For this review, take the finished solid that the model builds, in its own axes (mm). A direction names the side the tool comes from. Coordinates: 2 decimals unless noted, no trailing zeros. Write each loop counter-clockwise with the first axis right and the second up, starting at its lowest first coordinate (ties: lowest second). Pieces come first, ordered by that corner, then holes.
```python
from build123d import *

# Parameters (mm, degrees)
SKETCH1_W                      = 54
SKETCH1_H                      = 60
BOSS_EXTRUDE1_DEPTH            = 6
CBORE_FOR_M4_SHCS1_D           = 4.5
CBORE_FOR_M4_SHCS1_DEPTH       = 12.4
CBORE_FOR_M4_SHCS1_CBORE_D     = 8
CBORE_FOR_M4_SHCS1_CBORE_DEPTH = 4
CBORE_FOR_M4_SHCS1_TIP         = 1.351936393
CUT_EXTRUDE1_DEPTH             = 4
FILLET1_SIZE                   = 5
CUT_EXTRUDE2_DEPTH             = 41.804411681
BOSS_EXTRUDE2_START            = -5
SKETCH6_W                      = 14.857864376
SKETCH6_H                      = 14
SKETCH6_R                      = 3
BOSS_EXTRUDE2_DEPTH            = 36
FILLET3_SIZE                   = 5


with BuildPart() as part:
    # Sketch1 → Boss-Extrude1 (new body)
    with BuildSketch(Plane(origin=(0, 0, 0), x_dir=(1, 0, 0), z_dir=(0, 1, 0))):
        Rectangle(SKETCH1_W, SKETCH1_H)
    extrude(amount=BOSS_EXTRUDE1_DEPTH)

    # CBORE for M4 SHCS1
    with Locations(Plane(origin=(0, 6, 0), x_dir=(1, 0, 0), z_dir=(0, 1, 0))):
        with Locations((-22.5, 25.5), (-22.5, -25.5), (22.5, -25.5), (22.5, 25.5)):
            CounterBoreHole(CBORE_FOR_M4_SHCS1_D / 2, CBORE_FOR_M4_SHCS1_CBORE_D / 2, CBORE_FOR_M4_SHCS1_CBORE_DEPTH, depth=CBORE_FOR_M4_SHCS1_DEPTH)
            with Locations((0, 0, -(CBORE_FOR_M4_SHCS1_DEPTH + CBORE_FOR_M4_SHCS1_TIP / 2))):  # 118° drill point
                Cone(0, CBORE_FOR_M4_SHCS1_D / 2, CBORE_FOR_M4_SHCS1_TIP, mode=Mode.SUBTRACT)

    # Sketch4 → Cut-Extrude1 (cut)
    with BuildSketch(Plane(origin=(0, 6, 0), x_dir=(1, 0, 0), z_dir=(0, 1, 0))):
        with BuildLine():
            Line((-22.5, 21.5), (-27, 21.5))
            Line((-27, 21.5), (-27, 30))
            Line((-27, 30), (-18.5, 30))
            Line((-18.5, 30), (-18.5, 25.5))
            ThreePointArc((-18.5, 25.5), (-19.671572875, 22.671572875), (-22.5, 21.5))
        make_face()
        with BuildLine():
            Line((22.5, 21.5), (27, 21.5))
            Line((27, 21.5), (27, 30))
            Line((27, 30), (18.5, 30))
            Line((18.5, 30), (18.5, 25.5))
            ThreePointArc((18.5, 25.5), (19.671572875, 22.671572875), (22.5, 21.5))
        make_face()
        with BuildLine():
            Line((18.5, -30), (18.5, -25.5))
            ThreePointArc((18.5, -25.5), (19.671572875, -22.671572875), (22.5, -21.5))
            Line((22.5, -21.5), (27, -21.5))
            Line((27, -21.5), (27, -30))
            Line((27, -30), (18.5, -30))
        make_face()
        with BuildLine():
            Line((-18.5, -30), (-18.5, -25.5))
            ThreePointArc((-18.5, -25.5), (-19.671572875, -22.671572875), (-22.5, -21.5))
            Line((-22.5, -21.5), (-27, -21.5))
            Line((-27, -21.5), (-27, -30))
            Line((-27, -30), (-18.5, -30))
        make_face()
    extrude(amount=-CUT_EXTRUDE1_DEPTH, mode=Mode.SUBTRACT)

    # Fillet1
    # a fillet whose section is not a circle: 5 mm, written as the material it takes off along each edge
    with BuildSketch(Plane(origin=(27, -12.5, -30), x_dir=(0, 0, 1), z_dir=(0, 1, 0)), Plane(origin=(27, -12.5, 30), x_dir=(-1, 0, 0), z_dir=(0, 1, 0))) as fillet1_piece_1:
        with BuildLine():
            add(Edge.make_bspline([(FILLET1_SIZE, 0), (FILLET1_SIZE * 0.831801948466, 0), (FILLET1_SIZE * 0.663603896932, 0), (FILLET1_SIZE * 0.292893218813, -FILLET1_SIZE * 0.0716919198361), (FILLET1_SIZE * 0.0716919198361, -FILLET1_SIZE * 0.292893218813), (0, -FILLET1_SIZE * 0.663603896932), (0, -FILLET1_SIZE * 0.831801948466), (0, -FILLET1_SIZE)], knots=[0, 0, 0, 0, 0, 0, 0.5, 0.5, 1, 1, 1, 1, 1, 1], degree=5))
            Line((0, -FILLET1_SIZE), (0, 0))
            Line((0, 0), (FILLET1_SIZE, 0))
        make_face()
    extrude(amount=27, mode=Mode.SUBTRACT)
    with BuildSketch(Plane(origin=(-27, -12.5, -30), x_dir=(0, 0, 1), z_dir=(0, 1, 0)), Plane(origin=(-27, -12.5, 30), x_dir=(1, 0, 0), z_dir=(0, 1, 0))) as fillet1_piece_2:
        with BuildLine():
            add(Edge.make_bspline([(FILLET1_SIZE, 0), (FILLET1_SIZE * 0.831801948466, 0), (FILLET1_SIZE * 0.663603896932, 0), (FILLET1_SIZE * 0.292893218813, FILLET1_SIZE * 0.0716919198361), (FILLET1_SIZE * 0.0716919198361, FILLET1_SIZE * 0.292893218813), (0, FILLET1_SIZE * 0.663603896932), (0, FILLET1_SIZE * 0.831801948466), (0, FILLET1_SIZE)], knots=[0, 0, 0, 0, 0, 0, 0.5, 0.5, 1, 1, 1, 1, 1, 1], degree=5))
            Line((0, FILLET1_SIZE), (0, 0))
            Line((0, 0), (FILLET1_SIZE, 0))
        make_face()
    extrude(amount=27, mode=Mode.SUBTRACT)

    # Sketch5 → Cut-Extrude2 (cut, through all)
    with BuildSketch(Plane(origin=(0, 6, 0), x_dir=(1, 0, 0), z_dir=(0, 1, 0))):
        Polygon((-27, 13.5), (-23, 9.5), (-23, -9.5), (-27, -13.5), align=None)
        Polygon((27, 13.5), (23, 9.5), (23, -9.5), (27, -13.5), align=None)
    extrude(amount=-CUT_EXTRUDE2_DEPTH, mode=Mode.SUBTRACT)

    # Fillet2
    # a fillet whose section is not a circle: 5 mm, written as the material it adds along each edge
    with BuildSketch(Plane(origin=(-23, 6, 9.5), x_dir=(-0.7071067811865389, 0, 0.7071067811865561), z_dir=(0, -1, 0)), Plane(origin=(23, 6, 9.5), x_dir=(0, 0, -1), z_dir=(0, -1, 0)), Plane(origin=(23, 6, -9.5), x_dir=(0.707106781186557, 0, -0.7071067811865381), z_dir=(0, -1, 0)), Plane(origin=(-23, 6, -9.5), x_dir=(0, 0, 1), z_dir=(0, -1, 0))) as fillet2_piece_1:
        with BuildLine():
            add(Edge.make_bspline([(2.071067812, 0), (1.691961313, 0), (1.312854813, 0), (0.467093497, 0.07115949), (-0.279967621, 0.380602337), (-0.928328541, 0.928328541), (-1.196397318, 1.196397318), (-1.464466094, 1.464466094)], knots=[0, 0, 0, 0, 0, 0, 0.5, 0.5, 1, 1, 1, 1, 1, 1], degree=5))
            Line((-1.464466094, 1.464466094), (0, 0))
            Line((0, 0), (2.071067812, 0))
        make_face()
    extrude(amount=6)
    # a fillet whose section is not a circle: 5 mm, written as the material it takes off along each edge
    with BuildSketch(Plane(origin=(27, 11.17766953, 13.5), x_dir=(-0.7071067811865385, 0, -0.7071067811865565), z_dir=(0, -1, 0)), Plane(origin=(27, 11.17766953, -13.5), x_dir=(0, 0, -1), z_dir=(0, -1, 0)), Plane(origin=(-27, 11.17766953, 13.5), x_dir=(0, 0, 1), z_dir=(0, -1, 0)), Plane(origin=(-27, 11.17766953, -13.5), x_dir=(0.7071067811865569, 0, 0.707106781186538), z_dir=(0, -1, 0))) as fillet2_2_piece_1:
        with BuildLine():
            add(Edge.make_bspline([(2.071067812, 0), (1.691961313, 0), (1.312854813, 0), (0.467093497, -0.07115949), (-0.279967621, -0.380602337), (-0.928328541, -0.928328541), (-1.196397318, -1.196397318), (-1.464466094, -1.464466094)], knots=[0, 0, 0, 0, 0, 0, 0.5, 0.5, 1, 1, 1, 1, 1, 1], degree=5))
            Line((-1.464466094, -1.464466094), (0, 0))
            Line((0, 0), (2.071067812, 0))
        make_face()
    extrude(amount=16.355339059, mode=Mode.SUBTRACT)

    # Sketch6 → Boss-Extrude2 (add)
    with BuildSketch(Plane.ZY.offset(23).offset(BOSS_EXTRUDE2_START)):
        with Locations((0, 13)):
            Rectangle(SKETCH6_W, SKETCH6_H)
        with Locations((0, 14)):
            Circle(SKETCH6_R, mode=Mode.SUBTRACT)
    extrude(amount=-BOSS_EXTRUDE2_DEPTH)

    # Fillet3
    # a fillet whose section is not a circle: 5 mm, written as the material it takes off along each edge
    with BuildSketch(Plane(origin=(-30.5, 20, -7.428932188), x_dir=(0, -1, 0), z_dir=(1, 0, 0))) as fillet3_piece_1:
        with BuildLine():
            add(Edge.make_bspline([(FILLET3_SIZE, 0), (FILLET3_SIZE * 0.831801948466, 0), (FILLET3_SIZE * 0.663603896932, 0), (FILLET3_SIZE * 0.292893218813, -FILLET3_SIZE * 0.0716919198361), (FILLET3_SIZE * 0.0716919198361, -FILLET3_SIZE * 0.292893218813), (0, -FILLET3_SIZE * 0.663603896932), (0, -FILLET3_SIZE * 0.831801948466), (0, -FILLET3_SIZE)], knots=[0, 0, 0, 0, 0, 0, 0.5, 0.5, 1, 1, 1, 1, 1, 1], degree=5))
            Line((0, -FILLET3_SIZE), (0, 0))
            Line((0, 0), (FILLET3_SIZE, 0))
        make_face()
    extrude(amount=61, mode=Mode.SUBTRACT)
    with BuildSketch(Plane(origin=(-30.5, 20, 7.428932188), x_dir=(0, -1, 0), z_dir=(1, 0, 0))) as fillet3_piece_2:
        with BuildLine():
            add(Edge.make_bspline([(FILLET3_SIZE, 0), (FILLET3_SIZE * 0.831801948466, 0), (FILLET3_SIZE * 0.663603896932, 0), (FILLET3_SIZE * 0.292893218813, FILLET3_SIZE * 0.0716919198361), (FILLET3_SIZE * 0.0716919198361, FILLET3_SIZE * 0.292893218813), (0, FILLET3_SIZE * 0.663603896932), (0, FILLET3_SIZE * 0.831801948466), (0, FILLET3_SIZE)], knots=[0, 0, 0, 0, 0, 0, 0.5, 0.5, 1, 1, 1, 1, 1, 1], degree=5))
            Line((0, FILLET3_SIZE), (0, 0))
            Line((0, 0), (FILLET3_SIZE, 0))
        make_face()
    extrude(amount=61, mode=Mode.SUBTRACT)


solid = part.part
```
Q1. Add section B-B (z = 0). State the section outline as (x, y) points, then the cut area to 3 significant figures.
Ans:
outline: (-23, 0) - (23, 0) - (23, 6) - (18, 6) - (18, 11) - (-18, 11) - (-18, 6) - (-23, 6) - close; (-18, 17) - (18, 17) - (18, 20) - (-18, 20) - close
area: 564 mm2
Q2. Add section A-A (y = 14). State the section outline as (x, z) points, then the cut area to 3 significant figures.
Ans:
outline: (-18, -7.43) - (18, -7.43) - (18, -3) - (-18, -3) - close; (-18, 3) - (18, 3) - (18, 7.43) - (-18, 7.43) - close
area: 319 mm2
Q3. Tool access review of faces 1 (the flat face through (-18, 10, 0)), 2 (the flat face through (25, 4, -21.5)), 3 (the cylindrical face through (-19.703, 4.028, -22.641)): name each direction out of +Z, -Z, +X, -X, +Y, -Y from which nothing blocks a thin tool from reaching the whole face with its end or side.
Ans:
face 1: +Z, -Z, -X, +Y
face 2: -Z, +X, +Y
face 3: -Z, -X, +Y
Q4. Clearance check with flat-ended pins moving along their axes: pin 1 Ø8 at (x, z) = (1.5, -13) entering from +Y; pin 2 Ø4 at (y, z) = (7, 14.5) entering from +X; pin 3 Ø4 at (x, z) = (22.5, 25.5) entering from -Y; pin 4 Ø3 at (x, y) = (-25.5, 4) entering from -Z. State where each tip first meets the part, or that it passes through.
Ans:
pin 1: stops at y = 6
pin 2: stops at x = 27
pin 3: passes through
pin 4: stops at z = -21.5
Q5. Add section C-C (z = 22.5). State the section outline as (x, y) points, then the cut area to 3 significant figures.
Ans:
outline: (-27, 0) - (27, 0) - (27, 2) - (19.85, 2) - (19.85, 6) - (-19.85, 6) - (-19.85, 2) - (-27, 2) - close
area: 267 mm2
Q6. Draft analysis for pull direction X (two halves, no side actions). For faces 4 (the flat face through (18, 10, 0)), 5 (the flat face through (-27, 3, 19)), 6 (the cylindrical face through (-23.538, 0.986, 27.496)), 7 (the cylindrical face through (-23.538, 0.986, -23.504)), state which applies: +X half, -X half, draft (parallel to the pull), parting line (faces both ways), or undercut.
Ans:
face 4: +X half
face 5: -X half
face 6: undercut
face 7: undercut
Q7. Add section D-D (y = 7). State the section outline as (x, z) points.
Ans:
outline: (-18, -7.43) - (18, -7.43) - (18, 7.43) - (-18, 7.43) - close
Q8. For probe 1 along Z at (x, y) = (22.5, 1.5); probe 2 along X at (y, z) = (1.45, -25.5); probe 3 along Y at (x, z) = (-6, 0), list the stretches that pass through material, from the lowest coordinate up.
Ans:
probe 1: z = -30 to -27.75, -23.25 to 23.25, 27.75 to 30
probe 2: x = -27 to -24.75, -20.25 to 20.25, 24.75 to 27
probe 3: y = 0 to 11, 17 to 20
